Build history of the part. All positions in model axes, mm. Face numbers are marked on the shaded views. A direction names the side the tool comes from. Give positions to 0.01 mm unless a question says otherwise; leave off trailing zeros. Order: outer loops, then holes, each group sorted by start corner. A loop starts at its lowest first (then second) coordinate and runs counter-clockwise, first axis right, second up. Notation, with made-up numbers: M 18.25,-8 L 67.25,-8 A35 cw 67.25,27 Z; hole C 31,80.25 d10. An arc over 180 degrees is marked long. One line per item, written item: value.
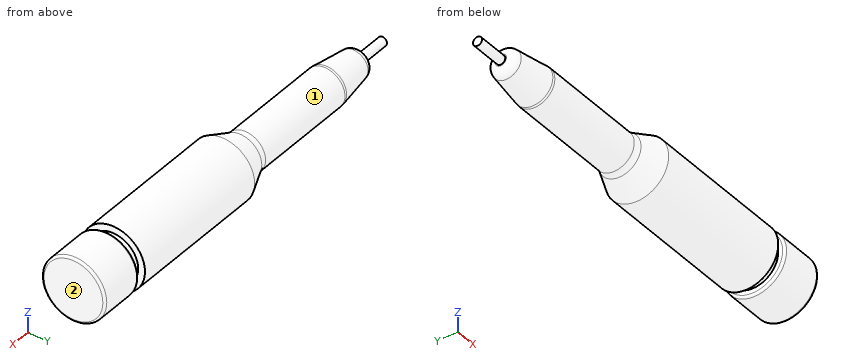
from build123d import *

# Parameters (mm, degrees)
FILETE1_R = 2
FILETE2_R = 4
FILETE3_R = 0.5


with BuildPart() as part:
    # Esboço1 → Revolução1 (revolve)
    with BuildSketch(Plane.XY):
        Polygon((0, 0), (0, 1), (7, 1), (7, 3), (17, 4.4), (42, 4.4), (48, 7), (81, 7), (81, 5.5), (83, 5.5), (83, 7), (93, 7), (93, 0), align=None)
    revolve(axis=Axis((93, 0, 0), (-1, 0, 0)))

    # Filete1
    filete1_edges = [part.edges().sort_by_distance(p)[0] for p in [
        (7, -3, 0),
    ]]
    fillet(filete1_edges, radius=FILETE1_R)

    # Filete2
    filete2_edges = [part.edges().sort_by_distance(p)[0] for p in [
        (42, -4.4, 0),
        (17, -4.4, 0),
    ]]
    fillet(filete2_edges, radius=FILETE2_R)

    # Filete3
    filete3_edges = [part.edges().sort_by_distance(p)[0] for p in [
        (93, -7, 0),
        (83, -7, 0),
    ]]
    fillet(filete3_edges, radius=FILETE3_R)


solid = part.part
1) Saw through at B-B, the plane x = 29. Write the cut outline in (y, z), then the cut area to 3 significant figures.
Check values:
outline: C 0,0 d8.8
area: 60.8 mm^2
2) Tool access for the marked faces 1 and 2: list every direction of +Z, -Z, +X, -X, +Y, -Y with a clear straight run to the whole face (end or side of a thin tool).
Check values:
face 1: -X
face 2: +Z, -Z, +X, +Y, -Y
3) Pin check, flat tips, straight feed: pin 1 (1.5 mm diameter, centred on x = 28.5, z = -4.5, fed in from +Y); pin 2 (1 mm diameter, centred on y = -4.5, z = 4.5, fed in from -X); pin 3 (6 mm diameter, centred on x = 82, z = -5.5, fed in from +Y). Stop position of each tip, or through.
Check values:
pin 1: y = 2.3
pin 2: x = 45.38
pin 3: y = 6.47
4) Drill centre lines: probe 1 along Y at (x, z) = (65, -0.25); probe 2 along Z at (x, y) = (34.5, -0.5); probe 3 along X at (y, z) = (-6, 1.5). Where is each one in solid material? Low to high. Write a range as from..to.
Check values:
probe 1: -7..7
probe 2: -4.37..4.37
probe 3: 46.12..81, 83..93
5) Saw through at A-A, the plane x = 73. Write the cut outline in (y, z).
Check values:
outline: C 0,0 d14
